Here's how the part is built. I have some questions about the finished solid (model axes, mm). A direction names the side the tool comes from. Give positions to 0.01 mm unless a question says otherwise; leave off trailing zeros. Write each loop counter-clockwise with the first axis right and the second up, starting at its lowest first coordinate (ties: lowest second). Pieces come first, ordered by that corner, then holes. Notation, with made-up numbers: (8.25, 53) -> (42.25, 53) arc R7 cw to (42.25, 64) -> close; hole circle Ø6 at (63.5, 85). An arc over 180 degrees is marked (long way). Return JSON: item names as keys, results as strings.
from build123d import *

# Parameters (mm, degrees)
BOSS_EXTRUDE1_DEPTH        = 25.4
SKETCH3_R                  = 3.81
CUT_EXTRUDE1_DEPTH         = 67.100379771
FILLET1_RADIUS             = 12.7
FILLET1_LENGTH             = 2.54
FILLET2_RADIUS             = 12.7
FILLET2_LENGTH             = 2.54
FILLET4_R                  = 19.05
FILLET5_RADIUS             = 21.59
FILLET5_LENGTH             = 25.4
FLATTEN_BENDS3_START       = 2.54
FLATTEN_BENDS3_OUTLINE_W   = 43.18
FLATTEN_BENDS3_OUTLINE_H   = 25.4
FLATTEN_BENDS3_DEPTH       = 38.1
FLATTEN_BENDS3_2_OUTLINE_W = 38.1
FLATTEN_BENDS3_2_OUTLINE_H = 25.4
FLATTEN_BENDS3_2_OUTLINE_R = 3.81
FLATTEN_BENDS3_2_DEPTH     = 2.54
PROCESS_BENDS3_DEPTH       = 25.4
PROCESS_BENDS3_2_OUTLINE_R = 3.81
PROCESS_BENDS3_2_DEPTH     = 2.54
PROCESS_BENDS3_3_DEPTH     = 25.4


# Read off the part's stored shape, not the designer's step: Flatten-Bends3, Process-Bends3
with BuildPart() as part:
    # Sketch2 → Boss-Extrude1 (new body)
    with BuildSketch(Plane.XY):
        Polygon((-43.375384615, 0), (-17.975384615, 0), (-17.975384615, 38.1), (20.124615385, 38.1), (20.124615385, 0), (45.524615385, 0), (45.524615385, 2.54), (22.664615385, 2.54), (22.664615385, 40.64), (-20.515384615, 40.64), (-20.515384615, 2.54), (-43.375384615, 2.54), align=None)
    extrude(amount=BOSS_EXTRUDE1_DEPTH)

    # Sketch3 → Cut-Extrude1 (cut, through all)
    with BuildSketch(Plane.XZ):
        with Locations(Location((-30.675384615, 12.7, 0), (0, 0, 270))):
            Circle(SKETCH3_R)
        with Locations(Location((32.824615385, 12.7, 0), (0, 0, 270))):
            Circle(SKETCH3_R)
    extrude(amount=-CUT_EXTRUDE1_DEPTH, mode=Mode.SUBTRACT)

    # Fillet1: full round fillet: the end face becomes a half cylinder, R = half its width
    fillet1_face = Plane((45.524615385, 1.27, 12.7), x_dir=(0, 1, 0), z_dir=(1, 0, 0))  # on the end face: x along it, z out of the body
    fillet1_slab = fillet1_face.offset(-FILLET1_RADIUS / 2) * Box(FILLET1_LENGTH, 2 * FILLET1_RADIUS, FILLET1_RADIUS, mode=Mode.PRIVATE)  # the body's end, R deep
    fillet1_round = Plane((32.824615385, 1.27, 12.7), x_dir=(1, 0, 0), z_dir=(0, 1, 0)) * Cylinder(FILLET1_RADIUS, FILLET1_LENGTH, mode=Mode.PRIVATE)  # its axis R under the face
    add(fillet1_slab - fillet1_round, mode=Mode.SUBTRACT)

    # Fillet2: full round fillet: the end face becomes a half cylinder, R = half its width
    fillet2_face = Plane((-43.375384615, 1.27, 12.7), x_dir=(0, -1, 0), z_dir=(-1, 0, 0))  # on the end face: x along it, z out of the body
    fillet2_slab = fillet2_face.offset(-FILLET2_RADIUS / 2) * Box(FILLET2_LENGTH, 2 * FILLET2_RADIUS, FILLET2_RADIUS, mode=Mode.PRIVATE)  # the body's end, R deep
    fillet2_round = Plane((-30.675384615, 1.27, 12.7), x_dir=(-1, 0, 0), z_dir=(0, -1, 0)) * Cylinder(FILLET2_RADIUS, FILLET2_LENGTH, mode=Mode.PRIVATE)  # its axis R under the face
    add(fillet2_slab - fillet2_round, mode=Mode.SUBTRACT)

    # Fillet4
    fillet4_edges = [part.edges().sort_by_distance(p)[0] for p in [
        (20.124615385, 38.1, 12.7),
        (-17.975384615, 38.1, 12.7),
    ]]
    fillet(fillet4_edges, radius=FILLET4_R - 0.0001)  # a hair under: the kernel refuses the full size

    # Fillet5: full round fillet: the end face becomes a half cylinder, R = half its width
    fillet5_face = Plane((1.074615385, 40.64, 12.7), x_dir=(0, 0, 1), z_dir=(0, 1, 0))  # on the end face: x along it, z out of the body
    fillet5_slab = fillet5_face.offset(-FILLET5_RADIUS / 2) * Box(FILLET5_LENGTH, 2 * FILLET5_RADIUS, FILLET5_RADIUS, mode=Mode.PRIVATE)  # the body's end, R deep
    fillet5_round = Plane((1.074615385, 19.05, 12.7), x_dir=(0, 1, 0), z_dir=(0, 0, 1)) * Cylinder(FILLET5_RADIUS, FILLET5_LENGTH, mode=Mode.PRIVATE)  # its axis R under the face
    add(fillet5_slab - fillet5_round, mode=Mode.SUBTRACT)

    # Flatten-Bends3 outline → Flatten-Bends3 (cut)
    with BuildSketch(Plane(origin=(0, 0, 0), x_dir=(1, 0, 0), z_dir=(0, 1, 0)).offset(FLATTEN_BENDS3_START)):
        with Locations((1.074615385, -12.7)):
            Rectangle(FLATTEN_BENDS3_OUTLINE_W, FLATTEN_BENDS3_OUTLINE_H)
    extrude(amount=FLATTEN_BENDS3_DEPTH, mode=Mode.SUBTRACT)

    # Flatten-Bends3 2 outline → Flatten-Bends3 2 (add)
    # profile 1 of 3: a face of its own
    with BuildSketch(Plane(origin=(0, 0, 0), x_dir=(1, 0, 0), z_dir=(0, 1, 0))):
        with Locations((1.074615385, -12.7)):
            Rectangle(FLATTEN_BENDS3_2_OUTLINE_W, FLATTEN_BENDS3_2_OUTLINE_H)
    # profile 2 of 3: a face of its own
    with BuildSketch(Plane(origin=(0, 0, 0), x_dir=(1, 0, 0), z_dir=(0, 1, 0))):
        with BuildLine():
            ThreePointArc((32.824615385, 0), (45.524615385, -12.7), (32.824615385, -25.4))
            Line((32.824615385, -25.4), (89.837494378, -25.4))
            ThreePointArc((89.837494378, -25.4), (102.537494378, -12.7), (89.837494378, 0))
            Line((89.837494378, 0), (32.824615385, 0))
        make_face()
        with Locations((89.837494378, -12.7)):
            Circle(FLATTEN_BENDS3_2_OUTLINE_R, mode=Mode.SUBTRACT)
    # profile 3 of 3: a face of its own
    with BuildSketch(Plane(origin=(0, 0, 0), x_dir=(1, 0, 0), z_dir=(0, 1, 0))):
        with Locations((32.824615385, -12.7)):
            Circle(FLATTEN_BENDS3_2_OUTLINE_R)
    extrude(amount=FLATTEN_BENDS3_2_DEPTH)

    # Process-Bends3 outline → Process-Bends3 (add)
    with BuildSketch(Plane.XY):
        with BuildLine():
            Line((22.664615385, 3.302), (22.664615385, 19.05))
            ThreePointArc((22.664615385, 19.05), (1.074615385, 40.64), (-20.515384615, 19.05))
            Line((-20.515384615, 19.05), (-20.515384615, 3.302))
            ThreePointArc((-20.515384615, 3.302), (-20.738569248, 2.763184633), (-21.277384615, 2.54))
            Line((-21.277384615, 2.54), (-18.064510513, 2.54))
            ThreePointArc((-18.064510513, 2.54), (-17.997741777, 2.918402742), (-17.975384615, 3.302))
            Line((-17.975384615, 3.302), (-17.975384615, 19.05))
            ThreePointArc((-17.975384615, 19.05), (1.074615385, 38.1), (20.124615385, 19.05))
            Line((20.124615385, 19.05), (20.124615385, 3.302))
            ThreePointArc((20.124615385, 3.302), (20.146972547, 2.918402742), (20.213741282, 2.54))
            Line((20.213741282, 2.54), (23.426615385, 2.54))
            ThreePointArc((23.426615385, 2.54), (22.887800018, 2.763184632), (22.664615385, 3.302))
        make_face()
    extrude(amount=PROCESS_BENDS3_DEPTH)

    # Process-Bends3 2 outline → Process-Bends3 2 (cut)
    # profile 1 of 2: a face of its own
    with BuildSketch(Plane(origin=(0, 0, 0), x_dir=(1, 0, 0), z_dir=(0, 1, 0))):
        with Locations((32.824615385, -12.7)):
            Circle(PROCESS_BENDS3_2_OUTLINE_R)
    # profile 2 of 2: a face of its own
    with BuildSketch(Plane(origin=(0, 0, 0), x_dir=(1, 0, 0), z_dir=(0, 1, 0))):
        with BuildLine():
            Line((89.837494378, 0), (32.824615385, 0))
            ThreePointArc((32.824615385, 0), (45.524615385, -12.7), (32.824615385, -25.4))
            Line((32.824615385, -25.4), (89.837494378, -25.4))
            ThreePointArc((89.837494378, -25.4), (102.537494378, -12.7), (89.837494378, 0))
        make_face()
        with Locations((89.837494378, -12.7)):
            Circle(PROCESS_BENDS3_2_OUTLINE_R, mode=Mode.SUBTRACT)
    extrude(amount=PROCESS_BENDS3_2_DEPTH, mode=Mode.SUBTRACT)

    # Process-Bends3 3 outline → Process-Bends3 3 (cut)
    with BuildSketch(Plane.XY):
        with BuildLine():
            ThreePointArc((23.426615385, 0), (21.378801917, 0.711698087), (20.213741282, 2.54))
            Line((20.213741282, 2.54), (-18.064510513, 2.54))
            ThreePointArc((-18.064510513, 2.54), (-19.229571147, 0.711698088), (-21.277384615, 0))
            Line((-21.277384615, 0), (23.426615385, 0))
        make_face()
    extrude(amount=PROCESS_BENDS3_3_DEPTH, mode=Mode.SUBTRACT)


solid = part.part
1. If I drill on line 1 (X direction, y = 15, z = 7.5); line 2 (X direction, y = 2, z = 12.7); line 3 (X direction, y = 1.95, z = 12.7), over which ranges is the centre line in solid material (lowest first)? Write a range as [from, to].
Taken from the geometry:
{"line 1": "x = [-20.52, -17.98], [20.12, 22.66]", "line 2": "x = [-43.38, -34.49], [-26.87, -18.24], [20.39, 29.01], [36.63, 45.52]", "line 3": "x = [-43.38, -34.49], [-26.87, -18.26], [20.41, 29.01], [36.63, 45.52]"}
2. Which directions (+Z, -Z, +X, -X, +Y, -Y) give clear straight access to the entire face, cutting with the end or side of a thin tool? Please do faces 5 (the face through (37, 2.54, 13)), 6 (the face through (20.125, 11, 13)), 7 (the face through (-20.515, 11, 13)).
Taken from the geometry:
{"face 5": "+Z, -Z, +X, +Y", "face 6": "+Z, -Z, -Y", "face 7": "+Z, -Z, -X, +Y"}
3. Suppose I cut it at D-D, the plane x = -8. List the corners of the cut face in (y, z) for me, and give its area (4 significant figures).
Taken from the geometry:
{"outline": "(35.8, 0) -> (38.64, 0) -> (38.64, 25.4) -> (35.8, 25.4) -> close", "area": "72.15 mm²"}
4. For pin 1 Ø8 at (x, z) = (33, 12.5) entering from +Y; pin 2 Ø12 at (y, z) = (31, 9.5) entering from -X; pin 3 Ø4 at (y, z) = (28, 9) entering from +X, each with a flat end and sliding along its axis, tell me the tip position at first contact or that it passes through.
Taken from the geometry:
{"pin 1": "stops at y = 2.54", "pin 2": "stops at x = -19.68", "pin 3": "stops at x = 21.52"}
5. Suppose I cut it at B-B, the plane z = 12.7. List the corners of the cut face in (x, y) for me.
Taken from the geometry:
{"outline": "(-43.38, 0) -> (-34.49, 0) -> (-34.49, 2.54) -> (-43.38, 2.54) -> close; (-26.87, 0) -> (-21.28, 0) arc R3.3 ccw to (-17.98, 3.3) -> (-17.98, 19.05) arc R19.05 cw to (20.12, 19.05) -> (20.12, 3.3) arc R3.3 ccw to (23.43, 0) -> (29.01, 0) -> (29.01, 2.54) -> (23.43, 2.54) arc R0.76 cw to (22.66, 3.3) -> (22.66, 19.05) arc R21.59 ccw to (-20.52, 19.05) -> (-20.52, 3.3) arc R0.76 cw to (-21.28, 2.54) -> (-26.87, 2.54) -> close; (36.63, 0) -> (45.52, 0) -> (45.52, 2.54) -> (36.63, 2.54) -> close"}
6. Suppose I cut it at A-A, the plane y = 9. List the corners of the cut face in (x, z) for me.
Taken from the geometry:
{"outline": "(-20.52, 0) -> (-17.98, 0) -> (-17.98, 25.4) -> (-20.52, 25.4) -> close; (20.12, 0) -> (22.66, 0) -> (22.66, 25.4) -> (20.12, 25.4) -> close"}
7. If we mould it in two halves opening along X, with no side actions, what happens to faces 1 (the face through (0.656, 38.095, 12.522)), 2 (the face through (-35, 0, 13)), 3 (the face through (32, 1.25, 16.42)), 4 (the face through (1.549, 40.635, 12.522))? For each: released by +X, released by -X, zero draft, split by the parting line, or undercut.
Taken from the geometry:
{"face 1": "undercut", "face 2": "zero draft", "face 3": "undercut", "face 4": "split by the parting line"}
8. Suppose I cut it at C-C, the plane z = 23.75. List the corners of the cut face in (x, y) for me.
Taken from the geometry:
{"outline": "(-36.94, 0) -> (-21.28, 0) arc R3.3 ccw to (-17.98, 3.3) -> (-17.98, 19.05) arc R19.05 cw to (20.12, 19.05) -> (20.12, 3.3) arc R3.3 ccw to (23.43, 0) -> (39.08, 0) -> (39.08, 2.54) -> (23.43, 2.54) arc R0.76 cw to (22.66, 3.3) -> (22.66, 19.05) arc R21.59 ccw to (-20.52, 19.05) -> (-20.52, 3.3) arc R0.76 cw to (-21.28, 2.54) -> (-36.94, 2.54) -> close"}
